Source: CAD feature listing. Evaluate the final solid. Frame: model axes, mm. A direction names the side the tool comes from. Coordinates: 2 decimals unless noted, no trailing zeros. Write each loop counter-clockwise with the first axis right and the second up, starting at its lowest first coordinate (ties: lowest second). Pieces come first, ordered by that corner, then holes. Notation, with made-up numbers: (-19, -30.75) -> (15, -30.75) arc R24 ccw to (15, -1.75) -> close; hole circle Ø8 at (-0.5, 70.5). An arc over 180 degrees is marked (long way). One line per item, written item: value. Start each with the question number.
1. Line query: line 1 (Y direction, x = 0, z = -2); line 2 (Y direction, x = 0, z = 14.75); line 3 (Z direction, x = 1.5, y = 11). Output: solid intervals per line, ascending.
2. Access query for faces 4 (the flat face through (0, 6, 25.4)), 5 (the cylindrical face through (-4.25, 5.07, -3.33)), 6 (the flat face through (5, 2, 0)). Directions: +Z, -Z, +X, -X, +Y, -Y. A direction counts if a zero-diameter tool reaches every point of the face in a straight line with its end or side. Return the directions, or none.
3. First-contact query: P1, Ø6, axis at x = 4, z = 8, coming from the +Y side; P2, Ø1, axis at y = 12, z = 5, coming from the +X side; P3, Ø2, axis at y = 6.18, z = -2.48, coming from the +X side. Flat tips, straight axial feed; report the tip coordinate or a pass-through.
4. Section query A-A, the plane y = 6.35. Output: boundary loops of the cut face in (x, z), and give its area (3 significant figures).
5. Mould query, pull axis Y, two halves, no side actions, for faces 1 (the conical face through (4.903, -3.076, 0.125)), 2 (the flat face through (3, 5, -5)), 3 (the flat face through (0, 6, 20)). Classes: released by +Y, released by -Y, zero draft, split by the parting line, or undercut.
6. Section query B-B, the plane z = 11.5. Output: boundary loops of the cut face in (x, y).
Autodesk Inventor part; units mm, degrees
ref_plane "YZ Plane" through (0, 0, 0) normal (1, 0, 0) x (0, 1, 0)
ref_plane "XZ Plane" through (0, 0, 0) normal (0, 1, 0) x (-1, 0, 0)
ref_plane "XY Plane" through (0, 0, 0) normal (0, 0, 1) x (1, 0, 0)
ref_plane "Work Plane1" through (0, 0, 0) normal (0, 0, 1) x (1, 0, 0)
sketch "Sketch1" plane through (0, 0, 0) normal (0, 0, 1) x (1, 0, 0)
  circle A0 centre (0, 6.35) radius 4
  circle A1 centre (0, 6.35) radius 12.5
  point P0 (0, 0)
  dimension "d0" = 25
extrude "Extrusion1" add sketch "Sketch1" along normal blind 25.4 contours A0 | A1
sketch "Skizze2" plane through (0, 6.35, 0) normal (0, 0, -1) x (-1, 0, 0)
  circle A0 centre (0, 0) radius 11
  circle A1 centre (0, 0) radius 2.9
  point P0 (0, -6.35)
  point P1 (-5.9, 11.95)
  dimension "d3" = 5.8
extrude "Extrusion2" cut sketch "Skizze2" against normal blind 20 contours A1
chamfer "Fase1" distance 2 angle 45 2 edges at (-12.5, 6.35, 25.4) (-12.5, 6.35, 0)
sketch "Skizze3" plane through (0, 6.35, 0) normal (0, 0, -1) x (-1, 0, 0)
  circle A0 centre (0, 0) radius 3
  circle A1 centre (0, 0) radius 2.9
  circle A2 centre (0, 0) radius 10.5
  circle A3 centre (0, 0) radius 6
  point P0 (0, -6.35)
  dimension "d9" = 12
extrude "Extrusion3" add sketch "Skizze3" along normal blind 5 contours A3
sketch "Skizze4" plane through (0, 0, 0) normal (1, 0, 0) x (0, 1, 0)
  circle A0 centre (6.1822, -2.4807) radius 1.4
  point P0 (0, 0)
  dimension "d12" = 2.8
extrude "Extrusion4" cut sketch "Skizze4" against normal through all
pattern_circular "Runde Anordnung1" count 3 over 360 about axis through (0, 6.35, 0) along (0, 0, -1) of "Extrusion4"
properties part number "ManualKnob"
Computed values:
1. line 1: y = 0.35 to 3.35, 9.35 to 12.35
1. line 2: y = -6.15 to 3.45, 9.25 to 18.85
1. line 3: z = -5 to -3.59, -1.37 to 25.4
2. face 4: +Z, +X, -X, +Y, -Y
2. face 5: -X
2. face 6: -Z
3. P1: stops at y = 18.81
3. P2: stops at x = 11.39
3. P3: stops at x = 6
4. outline: (-12.5, 2) -> (-10.5, 0) -> (-6, 0) -> (-6, -1.09) -> (-3, -1.09) -> (-3, 0) -> (-2.9, 0) -> (-2.9, 20) -> (2.9, 20) -> (2.9, 0) -> (3, 0) -> (3, -5) -> (6, -5) -> (6, 0) -> (10.5, 0) -> (12.5, 2) -> (12.5, 23.4) -> (10.5, 25.4) -> (-10.5, 25.4) -> (-12.5, 23.4) -> close; (-6, -5) -> (-3, -5) -> (-3, -3.87) -> (-6, -3.87) -> close
4. area: 533 mm²
5. face 1: split by the parting line
5. face 2: zero draft
5. face 3: undercut
6. outline: circle Ø25 at (0, 6.35); hole circle Ø5.8 at (0, 6.35)
